```python
from build123d import *

# Parameters (mm, degrees)
SKETCH1_W           = 50
SKETCH1_H           = 26
BOSS_EXTRUDE1_DEPTH = 18
SKETCH2_R           = 3.709825946
CUT_EXTRUDE1_DEPTH  = 3
FILLET1_R           = 5
CUT_EXTRUDE4_START  = -5
SKETCH3_W           = 7
SKETCH3_H           = 6
CUT_EXTRUDE4_DEPTH  = 5


with BuildPart() as part:
    # Sketch1 → Boss-Extrude1 (new body)
    with BuildSketch(Plane.XY):
        Rectangle(SKETCH1_W, SKETCH1_H)
    extrude(amount=BOSS_EXTRUDE1_DEPTH)

    # Sketch2 → Cut-Extrude1 (cut)
    with BuildSketch(Plane(origin=(25, 0, 0), x_dir=(0, 0, -1), z_dir=(1, 0, 0))):
        with Locations((-10.012439419, 5.395426064)):
            Circle(SKETCH2_R)
        Polygon((-10.012439419, -2.84865676), (-13.313646894, -4.754609784), (-13.313646894, -8.566515832), (-10.012439419, -10.472468856), (-6.711231945, -8.566515832), (-6.711231945, -4.754609784), align=None)
    extrude(amount=-CUT_EXTRUDE1_DEPTH, mode=Mode.SUBTRACT)

    # Fillet1
    fillet1_edges = [part.edges().sort_by_distance(p)[0] for p in [
        (0, -13, 18),
        (0, -13, 0),
        (0, 13, 0),
        (0, 13, 18),
    ]]
    fillet(fillet1_edges, radius=FILLET1_R)

    # Sketch3 → Cut-Extrude4 (cut)
    with BuildSketch(Plane.ZY.offset(25).offset(CUT_EXTRUDE4_START)):
        with BuildLine():
            Line((7, -4), (0, -4))
            Line((0, -4), (0, -8))
            ThreePointArc((0, -8), (0.105468435, -9.021548218), (0.417424305, -10))
            Line((0.417424305, -10), (7, -10))
            Line((7, -10), (7, -4))
        make_face()
        with Locations((3.5, -1)):
            Rectangle(SKETCH3_W, SKETCH3_H)
    extrude(amount=CUT_EXTRUDE4_DEPTH, mode=Mode.SUBTRACT)


solid = part.part
```
Geometry check sheet. Reference: the model listing, model coordinates, mm. A direction names the side the tool comes from. Coordinates: 2 decimals unless noted, no trailing zeros. Order: outer loops, then holes, each group sorted by start corner. A loop starts at its lowest first (then second) coordinate and runs counter-clockwise, first axis right, second up.
Q1. Sectioned sample at D-D on z = 12. Record the cut outline in (x, y), and give its area (3 significant figures).
Reply:
outline: (-25, -13) - (25, -13) - (25, -9.32) - (22, -9.32) - (22, -4) - (25, -4) - (25, 2.26) - (22, 2.26) - (22, 8.53) - (25, 8.53) - (25, 13) - (-25, 13) - close
area: 1,270 mm2
Q2. Tool access check on faces 1 (the face through (0, -13, 9)), 2 (the face through (-22, -4, 7)), 3 (the face through (23.52, 3.14, 12.96)). Record the directions out of +Z, -Z, +X, -X, +Y, -Y that give a thin tool (end or side, any length) a straight path to the whole face; none if there is none.
Reply:
face 1: +Z, -Z, +X, -X, -Y
face 2: -Z, -X
face 3: +X
Q3. Depth check by flat-ended pin: pin 1 Ø2 at (x, z) = (-5, 13.5) entering from -Y; pin 2 Ø3.5 at (y, z) = (6.5, 10) entering from +X; pin 3 Ø2 at (y, z) = (-3, 2) entering from -X; pin 4 Ø3 at (x, z) = (16.5, 16) entering from +Y. Enter the tip coordinate at first touch or a pass-through.
Reply:
pin 1: stops at y = -13
pin 2: stops at x = 22
pin 3: stops at x = -20
pin 4: stops at y = 12.77
Q4. Thickness scan on probe 1 along Z at (x, y) = (22.5, -6.25); probe 2 along X at (y, z) = (6, 8); probe 3 along X at (y, z) = (1.5, 6.25). Record the ranges inside material, lowest first.
Reply:
probe 1: z = 0 to 6.71, 13.31 to 18
probe 2: x = -25 to 22
probe 3: x = -20 to 25
Q5. Sectioned sample at A-A on y = -1.5. Record the cut outline in (x, z), and give its area (3 significant figures).
Reply:
outline: (-25, 7) - (-20, 7) - (-20, 0) - (25, 0) - (25, 18) - (-25, 18) - close
area: 865 mm2
Q6. Draft check along Y on faces 4 (the face through (0, -12, 16)), 5 (the face through (0, 0, 18)), 6 (the face through (24, -7, 13.314)), 7 (the face through (0, 13, 9)). Enter one of: released by +Y, released by -Y, zero draft, split by the parting line, or undercut.
Reply:
face 4: released by -Y
face 5: zero draft
face 6: undercut
face 7: released by +Y
Q7. Sectioned sample at B-B on x = 14. Record the cut outline in (y, z).
Reply:
outline: (-13, 5) arc R5 ccw to (-8, 0) - (8, 0) arc R5 ccw to (13, 5) - (13, 13) arc R5 ccw to (8, 18) - (-8, 18) arc R5 ccw to (-13, 13) - close
Q8. Sectioned sample at C-C on z = 8.5. Record the cut outline in (x, y).
Reply:
outline: (-25, -13) - (25, -13) - (25, -9.6) - (22, -9.6) - (22, -3.72) - (25, -3.72) - (25, 2.01) - (22, 2.01) - (22, 8.78) - (25, 8.78) - (25, 13) - (-25, 13) - close
